Verification items for the finished model (mm, model axes). Face numbers are marked on the shaded views. A direction names the side the tool comes from. Give positions to 0.01 mm unless a question says otherwise; leave off trailing zeros. Use one line per item in the form item = value. Start each with the question number.
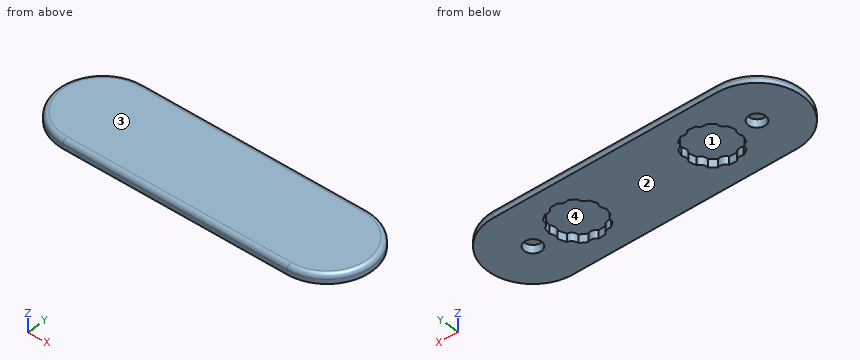
from build123d import *

# Parameters (mm, degrees)
PAD_DEPTH    = 2
FILLET_R     = 1
SKETCH001_R  = 1.9
POCKET_DEPTH = 1.82


with BuildPart() as part:
    # Sketch → Pad (new body)
    with BuildSketch(Plane.XY):
        with BuildLine():
            Line((-25.000026, 10), (25.000026, 10))
            ThreePointArc((25.000026, -10), (35, 0), (25.000026, 10))
            Line((25.000026, -10), (-25.000026, -10))
            ThreePointArc((-25.000026, 10), (-35, 0), (-25.000026, -10))
        make_face()
    extrude(amount=PAD_DEPTH)

    # Fillet
    fillet_edges = [part.edges().sort_by_distance(p)[0] for p in [
        (0, -10, 2),
        (-35, 0, 2),
        (0, 10, 2),
        (35, 0, 2),
    ]]
    fillet(fillet_edges, radius=FILLET_R)

    # Sketch001 → Pocket (cut)
    with BuildSketch(Plane.XY):
        with Locations((-25, 0)):
            Circle(SKETCH001_R)
        with Locations((25, 0)):
            Circle(SKETCH001_R)
        with BuildLine():
            ThreePointArc((-14.605792, 5.786588), (-13.752163, 5.202442), (-12.726434, 5.335813))
            Line((-12.726434, 5.335813), (-11.279808, 4.449738))
            ThreePointArc((-11.279808, 4.449738), (-10.93256, 3.475404), (-10.024334, 2.980395))
            Line((-10.024334, 2.980395), (-9.374811, 1.41324))
            ThreePointArc((-9.374811, 1.41324), (-9.666581, 0.42088), (-9.22277, -0.513433))
            Line((-9.22277, -0.513433), (-9.618445, -2.163068))
            ThreePointArc((-9.618445, -2.163068), (-10.437786, -2.794406), (-10.627911, -3.811147))
            Line((-11.91765, -4.913158), (-10.627911, -3.811147))
            ThreePointArc((-11.91765, -4.913158), (-12.951602, -4.942324), (-13.703041, -5.653132))
            Line((-15.394208, -5.786588), (-13.703041, -5.653132))
            ThreePointArc((-15.394208, -5.786588), (-16.247837, -5.202442), (-17.273566, -5.335813))
            Line((-18.720192, -4.449738), (-17.273566, -5.335813))
            ThreePointArc((-18.720192, -4.449738), (-19.06744, -3.475404), (-19.975666, -2.980395))
            Line((-20.625189, -1.41324), (-19.975666, -2.980395))
            ThreePointArc((-20.625189, -1.41324), (-20.333419, -0.42088), (-20.77723, 0.513433))
            Line((-20.381555, 2.163068), (-20.77723, 0.513433))
            ThreePointArc((-20.381555, 2.163068), (-19.562214, 2.794406), (-19.372089, 3.811147))
            Line((-19.372089, 3.811147), (-18.08235, 4.913158))
            ThreePointArc((-18.08235, 4.913158), (-17.048398, 4.942324), (-16.296959, 5.653132))
            Line((-16.296959, 5.653132), (-14.605792, 5.786588))
        make_face()
        with BuildLine():
            Line((20.648644, -1.316367), (20.026146, -2.894452))
            ThreePointArc((20.026146, -2.894452), (19.126561, -3.404995), (18.796108, -4.385153))
            Line((18.796108, -4.385153), (17.364922, -5.295956))
            ThreePointArc((17.364922, -5.295956), (16.337052, -5.180231), (15.493588, -5.778959))
            Line((15.493588, -5.778959), (13.800377, -5.674584))
            ThreePointArc((13.800377, -5.674584), (13.036835, -4.976794), (12.002534, -4.9654))
            Line((12.002534, -4.9654), (10.694048, -3.885714))
            ThreePointArc((10.694048, -3.885714), (10.48648, -2.872392), (9.65641, -2.255226))
            Line((9.65641, -2.255226), (9.232446, -0.612634))
            ThreePointArc((9.232446, -0.612634), (9.660136, 0.329167), (9.351356, 1.316367))
            Line((9.351356, 1.316367), (9.973854, 2.894452))
            ThreePointArc((9.973854, 2.894452), (10.873439, 3.404995), (11.203892, 4.385153))
            Line((11.203892, 4.385153), (12.635078, 5.295956))
            ThreePointArc((12.635078, 5.295956), (13.662948, 5.180231), (14.506412, 5.778959))
            Line((14.506412, 5.778959), (16.199623, 5.674584))
            ThreePointArc((16.199623, 5.674584), (16.963165, 4.976794), (17.997466, 4.9654))
            Line((17.997466, 4.9654), (19.305952, 3.885714))
            ThreePointArc((19.305952, 3.885714), (19.51352, 2.872392), (20.34359, 2.255226))
            Line((20.34359, 2.255226), (20.767554, 0.612634))
            ThreePointArc((20.767554, 0.612634), (20.339864, -0.329167), (20.648644, -1.316367))
        make_face()
    extrude(amount=POCKET_DEPTH, mode=Mode.SUBTRACT)


solid = part.part
Item 1: Sectioned sample at A-A, the plane z = 0.7. State how many separate pieces and enclosed holes the cut face has, and give its area (3 significant figures).
Item 2: Tool access check on the marked faces 3 and 4. Record the directions out of +Z, -Z, +X, -X, +Y, -Y that give a thin tool (end or side, any length) a straight path to the whole face; none if there is none.
Item 3: Draft check along Y on the marked faces 1 and 2. Enter one of: +Y half, -Y half, draft (parallel to the pull), parting line (faces both ways), or undercut.
Item 4: Material ranges on line 1 (Y direction, x = 25, z = 0.5); line 2 (X direction, y = -5, z = 0.75); line 3 (X direction, y = -0.25, z = 1.15), recorded low to high.
Item 5: Gauge pin test, flat end, axial feed: pin 1 Ø1.1 at (x, y) = (25, 0) entering from -Z. Record the tip position at first contact, or that the pin passes through.
Outcome:
q1.separate_pieces = 1
q1.enclosed_holes = 4
q1.area = 1,090 mm^2
q2.face_3 = +Z, +X, -X, +Y, -Y
q2.face_4 = -Z
q3.face_1 = undercut
q3.face_2 = draft
q4.line_1 = -10 to -1.9, 1.9 to 10
q4.line_2 = -33.66 to -17.82, -13.07 to 13.09, 17.83 to 33.66
q4.line_3 = -34.99 to -26.88, -23.12 to -20.36, -9.44 to 9.5, 20.35 to 23.12, 26.88 to 34.99
q5.pin_1 = 1.82
